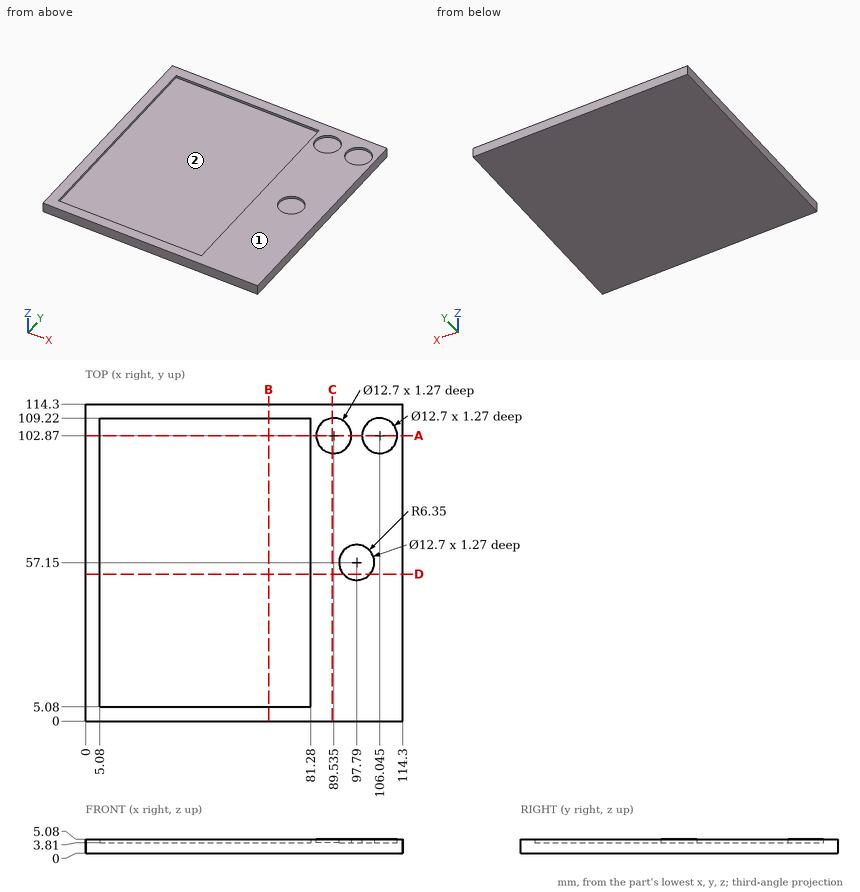
The drawing under review shows one solid part. Ordinate dimensions are in mm from its lowest x, y, z. Coordinates: 2 decimals unless noted, no trailing zeros. Loops run counter-clockwise (first coordinate to the right, second up) from the corner with the lowest first, then second, coordinate; pieces in that order, holes last. Notation, with made-up numbers: (51, 30.25) -> (77, 30.25) arc R31 ccw to (77, 61.25) -> close; hole circle Ø6 at (26.25, 85). An arc over 180 degrees is marked (long way). Answer as a JSON object with one key per item and string values.
Q1. Take a section at A-A on y = 102.87. Give the boundary of the cut face in (x, z) (3 decimals).
Answer block:
{"outline": "(0, 0) -> (114.3, 0) -> (114.3, 5.08) -> (112.395, 5.08) -> (112.395, 3.81) -> (99.695, 3.81) -> (99.695, 5.08) -> (95.885, 5.08) -> (95.885, 3.81) -> (83.185, 3.81) -> (83.185, 5.08) -> (81.28, 5.08) -> (81.28, 3.81) -> (5.08, 3.81) -> (5.08, 5.08) -> (0, 5.08) -> close"}
Q2. The part is to be moulded in two halves that separate along Y. For the marked faces 1 and 2, say which applies: +Y half, -Y half, draft (parallel to the pull), parting line (faces both ways), or undercut.
Answer block:
{"face 1": "draft", "face 2": "undercut"}
Q3. To check wall thickness, follow L1, parallel to X at y = 57.15, z = 4.6; L2, parallel to Y at x = 16.5, z = 4.95; L3, parallel to X at y = 67.5, z = 4.85. State the ranges of each line that lie inside material, in increasing order.
Answer block:
{"L1": "x = 0 to 5.08, 81.28 to 91.44, 104.14 to 114.3", "L2": "y = 0 to 5.08, 109.22 to 114.3", "L3": "x = 0 to 5.08, 81.28 to 114.3"}
Q4. Take a section at D-D on y = 53. Give the boundary of the cut face in (x, z), plus the area to 3 significant figures.
Answer block:
{"outline": "(0, 0) -> (114.3, 0) -> (114.3, 5.08) -> (102.6, 5.08) -> (102.6, 3.81) -> (92.98, 3.81) -> (92.98, 5.08) -> (81.28, 5.08) -> (81.28, 3.81) -> (5.08, 3.81) -> (5.08, 5.08) -> (0, 5.08) -> close", "area": "472 mm^2"}
Q5. Take a section at B-B on x = 66. Give the boundary of the cut face in (y, z), plus the area to 3 significant figures.
Answer block:
{"outline": "(0, 0) -> (114.3, 0) -> (114.3, 5.08) -> (109.22, 5.08) -> (109.22, 3.81) -> (5.08, 3.81) -> (5.08, 5.08) -> (0, 5.08) -> close", "area": "448 mm^2"}
Q6. Take a section at C-C on x = 89. Give the boundary of the cut face in (y, z).
Answer block:
{"outline": "(0, 0) -> (114.3, 0) -> (114.3, 5.08) -> (109.2, 5.08) -> (109.2, 3.81) -> (96.54, 3.81) -> (96.54, 5.08) -> (0, 5.08) -> close"}
Q7. Clearance check with flat-ended pins moving along their axes: pin 1 Ø14.5 at (x, y) = (106.045, 102.87) entering from -Z; pin 2 Ø3 at (x, y) = (76, 96.5) entering from +Z. State where each tip first meets the part, or that it passes through.
Answer block:
{"pin 1": "stops at z = 0", "pin 2": "stops at z = 3.81"}
